Model file for the job. Use its own axes, mm. Face numbers are marked on the shaded views. A direction names the side the tool comes from. Round coordinates to 2 decimals unless told otherwise and drop trailing zeros. Write each loop counter-clockwise with the first axis right and the second up, starting at its lowest first coordinate (ties: lowest second). Pieces come first, ordered by that corner, then holes. Notation, with made-up numbers: (-39.75, 16) - (-11.75, 16) arc R31 cw to (-11.75, 53) - close; hole circle Ø4 at (-17, 14). An arc over 180 degrees is marked (long way). One line per item, written item: value.
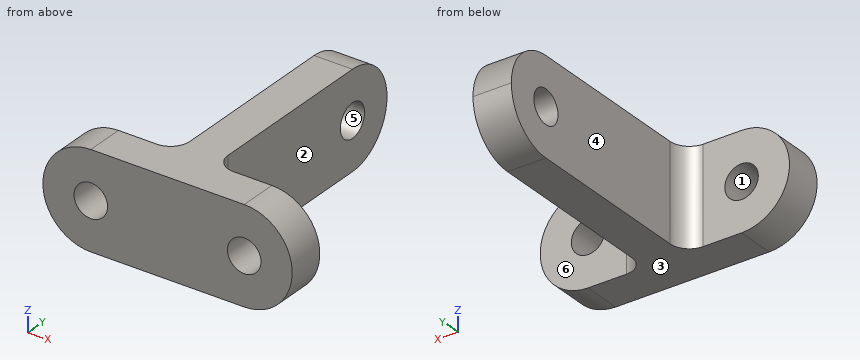
from build123d import *

# Parameters (mm, degrees)
SKETCH1_R           = 5
SKETCH1_R_2         = 1.75
BOSS_EXTRUDE1_DEPTH = 4
SKETCH2_W           = 4
SKETCH2_H           = 10
BOSS_EXTRUDE2_DEPTH = 25
SKETCH3_R           = 1.75
CUT_EXTRUDE1_DEPTH  = 4
FILLET1_R           = 2
FILLET2_R           = 2


with BuildPart() as part:
    # Sketch1 → Boss-Extrude1 (new body)
    # profile 1 of 3: a face of its own
    with BuildSketch(Plane(origin=(0, 0, 0), x_dir=(1, 0, 0), z_dir=(0, 1, 0))):
        with Locations((-8, 0)):
            Circle(SKETCH1_R)
        with Locations(Location((-8, 0, 0), (0, 0, 270))):
            Circle(SKETCH1_R_2, mode=Mode.SUBTRACT)
    # profile 2 of 3: a face of its own
    with BuildSketch(Plane(origin=(0, 0, 0), x_dir=(1, 0, 0), z_dir=(0, 1, 0))):
        with BuildLine():
            Line((8, 5), (-8, 5))
            ThreePointArc((-8, 5), (-4.464466094, 3.535533906), (-3, 0))
            ThreePointArc((-3, 0), (-4.464466094, -3.535533906), (-8, -5))
            Line((-8, -5), (8, -5))
            ThreePointArc((8, -5), (3, 0), (8, 5))
        make_face()
    # profile 3 of 3: a face of its own
    with BuildSketch(Plane(origin=(0, 0, 0), x_dir=(1, 0, 0), z_dir=(0, 1, 0))):
        with Locations((8, 0)):
            Circle(SKETCH1_R)
        with Locations(Location((8, 0, 0), (0, 0, 270))):
            Circle(SKETCH1_R_2, mode=Mode.SUBTRACT)
    extrude(amount=BOSS_EXTRUDE1_DEPTH)

    # Sketch2 → Boss-Extrude2 (add)
    with BuildSketch(Plane(origin=(0, 4, 0), x_dir=(1, 0, 0), z_dir=(0, 1, 0))):
        Rectangle(SKETCH2_W, SKETCH2_H)
    extrude(amount=BOSS_EXTRUDE2_DEPTH)

    # Sketch3 → Cut-Extrude1 (cut)
    with BuildSketch(Plane(origin=(2, 0, 0), x_dir=(0, 0, -1), z_dir=(1, 0, 0))):
        with BuildLine():
            Line((-5, 29), (-5, 24))
            ThreePointArc((-5, 24), (-3.535533915, 27.535533897), (-2.5e-08, 29))
            Line((-2.5e-08, 29), (-5, 29))
        make_face()
        with BuildLine():
            ThreePointArc((-2.5e-08, 29), (3.535533897, 27.535533915), (5, 24))
            Line((5, 24), (5, 29))
            Line((5, 29), (-2.5e-08, 29))
        make_face()
        with Locations((0, 24)):
            Circle(SKETCH3_R)
    extrude(amount=-CUT_EXTRUDE1_DEPTH, mode=Mode.SUBTRACT)

    # Fillet1
    fillet1_edges = [part.edges().sort_by_distance(p)[0] for p in [
        (2, 4, 0),
    ]]
    fillet(fillet1_edges, radius=FILLET1_R)

    # Fillet2
    fillet2_edges = [part.edges().sort_by_distance(p)[0] for p in [
        (-2, 4, 0),
    ]]
    fillet(fillet2_edges, radius=FILLET2_R)


solid = part.part
1. Tool access for the marked faces 4, 5 and 6: list every direction of +Z, -Z, +X, -X, +Y, -Y with a clear straight run to the whole face (end or side of a thin tool).
Report:
face 4: +Z, -Z, -X, +Y
face 5: +X, -X
face 6: +Z, -Z, +X, +Y
2. Band-saw the part on D-D on y = 23. Write the cut outline in (x, z).
Report:
outline: (-2, -5) - (2, -5) - (2, -1.44) - (-2, -1.44) - close; (-2, 1.44) - (2, 1.44) - (2, 5) - (-2, 5) - close
3. Band-saw the part on C-C on z = -3. Write the cut outline in (x, y).
Report:
outline: (-12, 0) - (12, 0) - (12, 4) - (4, 4) arc R2 cw to (2, 6) - (2, 28) - (-2, 28) - (-2, 6) arc R2 cw to (-4, 4) - (-12, 4) - close
4. Band-saw the part on A-A on z = 1.25. Write the cut outline in (x, y), plus the area to 3 significant figures.
Report:
outline: (-12.84, 0) - (-9.22, 0) - (-9.22, 4) - (-12.84, 4) - close; (-6.78, 0) - (6.78, 0) - (6.78, 4) - (4, 4) arc R2 cw to (2, 6) - (2, 22.78) - (-2, 22.78) - (-2, 6) arc R2 cw to (-4, 4) - (-6.78, 4) - close; (-2, 25.22) - (2, 25.22) - (2, 28.84) - (-2, 28.84) - close; (9.22, 0) - (12.84, 0) - (12.84, 4) - (9.22, 4) - close
area: 174 mm²
5. Wall check: probe 1 along X at (y, z) = (1, 0); probe 2 along X at (y, z) = (17.75, 1.5); probe 3 along Y at (x, z) = (6.25, -2.25). Give the ranges that are in metal, low to high. Write a range as [from, to].
Report:
probe 1: [-13, -9.75], [-6.25, 6.25], [9.75, 13]
probe 2: [-2, 2]
probe 3: [0, 4]
6. Band-saw the part on B-B on x = -7. Write the cut outline in (y, z), plus the area to 3 significant figures.
Report:
outline: (0, -5) - (4, -5) - (4, -1.44) - (0, -1.44) - close; (0, 1.44) - (4, 1.44) - (4, 5) - (0, 5) - close
area: 28.5 mm²
7. Drop flat-ended pins along their axis: pin 1 (5 mm diameter, centred on y = 22.5, z = 2, fed in from +X); pin 2 (6 mm diameter, centred on x = 4, y = 12.5, fed in from -Z); pin 3 (2.5 mm diameter, centred on x = -10.5, z = -0.5, fed in from +Y); pin 4 (5 mm diameter, centred on y = 12.5, z = 0.5, fed in from -X). Give the stop position or say it passes through.
Report:
pin 1: x = 2
pin 2: z = -5
pin 3: y = 4
pin 4: x = -2
8. Mould opens along Z. For the marked faces 1, 2 and 3 say: released by +Z, released by -Z, zero draft, split by the parting line, or undercut.
Report:
face 1: undercut
face 2: zero draft
face 3: released by -Z
